Geometry check sheet. Reference: drawing and pictorial views, mm from the part's lowest x, y, z. Round coordinates to 2 decimals unless told otherwise and drop trailing zeros. Write each loop counter-clockwise with the first axis right and the second up, starting at its lowest first coordinate (ties: lowest second). Pieces come first, ordered by that corner, then holes. Notation, with made-up numbers: (23.25, 75.25) -> (79.25, 75.25) arc R31 cw to (79.25, 102.25) -> close; hole circle Ø1 at (-23.5, -23.75). An arc over 180 degrees is marked (long way). Answer as a JSON object with one key per item and string values. Group by question number.
(1) Sectioned sample at A-A on y = 117. Record the cut outline in (x, z).
(2) Sectioned sample at C-C on y = 580. Record the cut outline in (x, z).
(3) Scan lines: L1, parallel to Y at x = 17.5, z = 628; L2, parallel to Z at x = 19, y = 412; L3, parallel to Y at x = 18.75, z = 854.5. Record each from-to range of solid material in increasing order. Write a range as from..to.
(4) Sectioned sample at B-B on x = 5.25. Record the cut outline in (y, z), and give its area (3 significant figures).
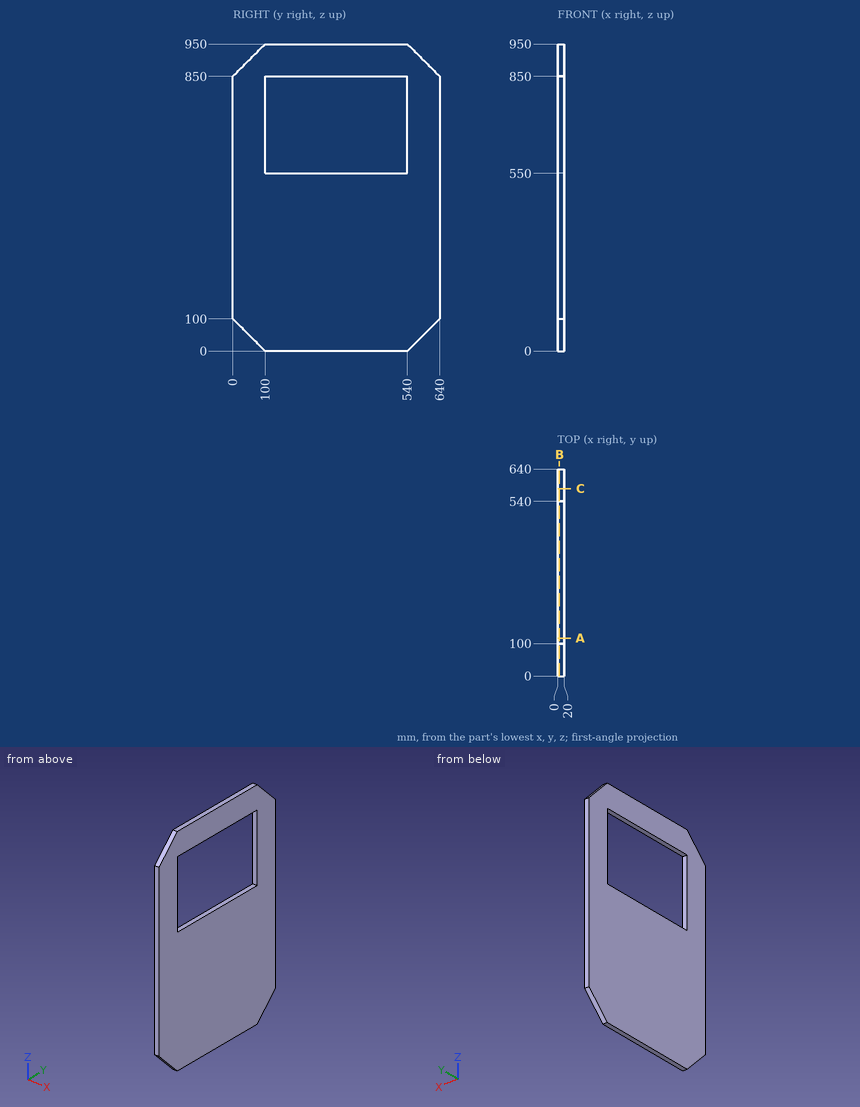
Computed values:
{
 "1": {"outline": "(0, 0) -> (20, 0) -> (20, 550) -> (0, 550) -> close; (0, 850) -> (20, 850) -> (20, 950) -> (0, 950) -> close"},
 "2": {"outline": "(0, 40) -> (20, 40) -> (20, 910) -> (0, 910) -> close"},
 "3": {"L1": "0..100, 540..640", "L2": "0..550, 850..950", "L3": "4.5..635.5"},
 "4": {"outline": "(0, 100) -> (100, 0) -> (540, 0) -> (640, 100) -> (640, 850) -> (540, 950) -> (100, 950) -> (0, 850) -> close; hole (100, 550) -> (540, 550) -> (540, 850) -> (100, 850) -> close", "area": "456,000 mm2"}
}
